Check sheet for the modelled part. Datum: model origin and axes. Units: mm. A direction names the side the tool comes from. Coordinates: 2 decimals unless noted, no trailing zeros. Loops run counter-clockwise (first coordinate to the right, second up) from the corner with the lowest first, then second, coordinate; pieces in that order, holes last. Notation, with made-up numbers: M -12,58.25 L 46,58.25 A11 ccw 46,66.25 Z; hole C 37.5,-31.75 d9. An arc over 180 degrees is marked long. Use CSV: the item, a comma, the result in double quotes. Start each with the question number.
(1) Go/stop test with flat-tipped pins: pin 1 Ø10 at (y, z) = (-3.5, 28.5) entering from -X; pin 2 Ø1.5 at (y, z) = (-5.5, 26) entering from -X; pin 3 Ø3 at (x, z) = (-2, 53) entering from -Y. Record where each tip stops, or that it passes through.
(2) Draft check along Z on faces 1 (the flat face through (-3, -13, 63)), 2 (the flat face through (-4, -12, 0)), 3 (the flat face through (-13, -17, 32)). Enter one of: pulls with the +Z half, pulls with the -Z half, needs draft (parallel to the pull), parting line crosses it, or undercut.
(3) Section check A-A on y = -7.5. Record the cut outline in (x, z), and give its area (3 significant figures).
(4) Set-up check for faces 4 (the flat face through (0, -1.5, 32.3)), 5 (the flat face through (-6.31, -9.55, 32.07)): record each of +Z, -Z, +X, -X, +Y, -Y from which the full face is reachable in a straight line by a thin tool's end or side.
(5) Section check B-B on x = -3. Record the cut outline in (y, z).
(6) Section check C-C on z = 35. Record the cut outline in (x, y).
(7) Scan lines: line 1 (Z direction, x = -0.75, y = -14.75); line 2 (X direction, y = -12.5, z = 60.5); line 3 (X direction, y = -13.5, z = 51). Record each from-to range of solid material in increasing order.
from build123d import *

# Parameters (mm, degrees)
BOSS_EXTRUDE2_DEPTH = 2
BOSS_EXTRUDE3_DEPTH = 61
BOSS_EXTRUDE4_DEPTH = 2


with BuildPart() as part:
    # Sketch1 → Boss-Extrude2 (new body)
    with BuildSketch(Plane.XY):
        Polygon((0, 0), (0, -17), (-14, -17), align=None)
    extrude(amount=BOSS_EXTRUDE2_DEPTH)

    # Sketch5 → Boss-Extrude3 (add)
    with BuildSketch(Plane.XY.offset(2)):
        Polygon((-14, -17), (-12.445455373, -17), (0, -1.887661332), (0, 0), align=None)
    extrude(amount=BOSS_EXTRUDE3_DEPTH)

    # Sketch6 → Boss-Extrude4 (add)
    with BuildSketch(Plane.XY.offset(63)):
        Polygon((0, 0), (0, -17), (-14, -17), align=None)
    extrude(amount=BOSS_EXTRUDE4_DEPTH)


solid = part.part
Outcome:
1,pin 1,"stops at x = -7"
1,pin 2,"stops at x = -5.15"
1,pin 3,"stops at y = -6.14"
2,face 1,"undercut"
2,face 2,"pulls with the -Z half"
2,face 3,"needs draft"
3,outline,"M -6.18,0 L 0,0 L 0,2 L -4.62,2 L -4.62,63 L 0,63 L 0,65 L -6.18,65 Z"
3,area,"120 mm²"
4,face 4,"+Z, -Z, +X, +Y, -Y"
4,face 5,"+X, -Y"
5,outline,"M -17,0 L -3.64,0 L -3.64,65 L -17,65 L -17,63 L -5.53,63 L -5.53,2 L -17,2 Z"
6,outline,"M -14,-17 L -12.45,-17 L 0,-1.89 L 0,0 Z"
7,line 1,"z = 0 to 2, 63 to 65"
7,line 2,"x = -10.29 to -8.74"
7,line 3,"x = -11.12 to -9.56"
